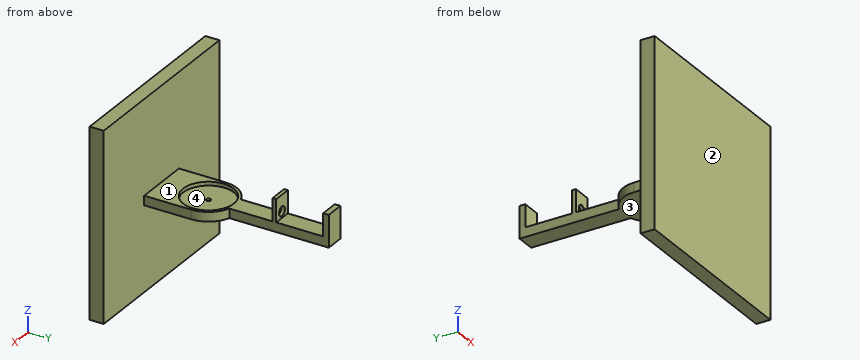
```python
from build123d import *

# Parameters (mm, degrees)
SKETCH1_W           = 100
SKETCH1_H           = 7.5
BOSS_EXTRUDE1_DEPTH = 100
BOSS_EXTRUDE2_START = 45
BOSS_EXTRUDE2_DEPTH = 5
SKETCH3_R           = 13.5
CUT_EXTRUDE1_DEPTH  = 2
SKETCH4_W           = 10
SKETCH4_H           = 3
BOSS_EXTRUDE3_DEPTH = 17
SKETCH6_W           = 10
SKETCH6_H           = 12
SKETCH6_R           = 2.5
BOSS_EXTRUDE4_DEPTH = 2
CUT_EXTRUDE2_REACH  = 152.441
SKETCH7_R           = 1.25


with BuildPart() as part:
    # Sketch1 → Boss-Extrude1 (new body)
    with BuildSketch(Plane.XY):
        with Locations((50, 3.75)):
            Rectangle(SKETCH1_W, SKETCH1_H)
    extrude(amount=BOSS_EXTRUDE1_DEPTH)

    # Sketch2 → Boss-Extrude2 (add)
    with BuildSketch(Plane.XY.offset(BOSS_EXTRUDE2_START)):
        with BuildLine():
            Line((35, 7.5), (65, 7.5))
            Line((65, 7.5), (65, 32.5))
            ThreePointArc((65, 32.5), (62.247448714, 41.160254038), (55, 46.642135624))
            Line((55, 46.642135624), (55, 96.642135624))
            Line((55, 96.642135624), (45, 96.642135624))
            Line((45, 96.642135624), (45, 46.642135624))
            ThreePointArc((45, 46.642135624), (37.752551286, 41.160254038), (35, 32.5))
            Line((35, 32.5), (35, 7.5))
        make_face()
    extrude(amount=BOSS_EXTRUDE2_DEPTH)

    # Sketch3 → Cut-Extrude1 (cut)
    with BuildSketch(Plane.XY.offset(50)):
        with Locations((50, 32.5)):
            Circle(SKETCH3_R)
    extrude(amount=-CUT_EXTRUDE1_DEPTH, mode=Mode.SUBTRACT)

    # Sketch4 → Boss-Extrude3 (add)
    with BuildSketch(Plane(origin=(0, 0, 45), x_dir=(-1, 0, 0), z_dir=(0, 0, -1))):
        with Locations((-50, 98.142135624)):
            Rectangle(SKETCH4_W, SKETCH4_H)
    extrude(amount=-BOSS_EXTRUDE3_DEPTH)

    # Sketch6 → Boss-Extrude4 (add)
    with BuildSketch(Plane(origin=(0, 71.642135624, 0), x_dir=(-1, 0, 0), z_dir=(0, -1, 0))):
        with Locations((-50, -56)):
            Rectangle(SKETCH6_W, SKETCH6_H)
        with Locations(Location((-50, -53.5, 0), (0, 0, 90))):
            Circle(SKETCH6_R, mode=Mode.SUBTRACT)
    extrude(amount=BOSS_EXTRUDE4_DEPTH)

    # Sketch7 → Cut-Extrude2 (cut, up to next)
    with BuildSketch(Plane.XY.offset(48), mode=Mode.PRIVATE) as cut_extrude2_sk1:
        with Locations((50, 32.5)):
            Circle(SKETCH7_R)
    cut_extrude2_tool1 = extrude(cut_extrude2_sk1.sketch, amount=-CUT_EXTRUDE2_REACH, mode=Mode.PRIVATE) & part.part
    add(cut_extrude2_tool1.solids().sort_by_distance((50, 32.5, 48))[0], mode=Mode.SUBTRACT)


solid = part.part
```
Build history of the part. All positions in model axes, mm. Face numbers are marked on the shaded views. Round coordinates to 2 decimals unless told otherwise and drop trailing zeros. Write each loop counter-clockwise with the first axis right and the second up, starting at its lowest first coordinate (ties: lowest second). Pieces come first, ordered by that corner, then holes.
1) Band-saw the part on D-D, the plane x = 93.5. List the corners of the cut face in (y, z).
2) Pin check, flat tips, straight feed: pin 1 (5.5 mm diameter, centred on y = 25, z = 46.5, fed in from +X); pin 2 (1.5 mm diameter, centred on y = 41.5, z = 47.5, fed in from +X); pin 3 (11 mm diameter, centred on x = 50, y = 87.5, fed in from +Z). Stop position of each tip, or through.
3) Band-saw the part on C-C, the plane y = 54.5. List the corners of the cut face in (x, z).
4) Drill centre lines: probe 1 along Y at (x, z) = (50, 45.6); probe 2 along Y at (x, z) = (62, 56); probe 3 along X at (y, z) = (70.15, 53.5). Where is each one in solid material? Low to high.
5) Band-saw the part on A-A, the plane z = 53.5. List the corners of the cut face in (x, y).
6) Mould opens along Y. For the marked faces 1, 2, 3 and 4 say: +Y half, -Y half, draft (parallel to the pull), parting line (faces both ways), or undercut.
7) Band-saw the part on B-B, the plane x = 61. List the corners of the cut face in (y, z).
Ans:
1. outline: (0, 0) - (7.5, 0) - (7.5, 100) - (0, 100) - close
2. pin 1: stops at x = 65
2. pin 2: stops at x = 62.53
2. pin 3: stops at z = 50
3. outline: (45, 45) - (55, 45) - (55, 50) - (45, 50) - close
4. probe 1: y = 0 to 31.25, 33.75 to 99.64
4. probe 2: y = 0 to 7.5
4. probe 3: x = 45 to 47.5, 52.5 to 55
5. outline: (0, 0) - (100, 0) - (100, 7.5) - (0, 7.5) - close; (45, 69.64) - (47.5, 69.64) - (47.5, 71.64) - (45, 71.64) - close; (45, 96.64) - (55, 96.64) - (55, 99.64) - (45, 99.64) - close; (52.5, 69.64) - (55, 69.64) - (55, 71.64) - (52.5, 71.64) - close
6. face 1: undercut
6. face 2: -Y half
6. face 3: draft
6. face 4: undercut
7. outline: (0, 0) - (7.5, 0) - (7.5, 45) - (42.7, 45) - (42.7, 50) - (40.33, 50) - (40.33, 48) - (24.67, 48) - (24.67, 50) - (7.5, 50) - (7.5, 100) - (0, 100) - close
